Build history of the part. All positions in model axes, mm. A direction names the side the tool comes from. Give positions to 0.01 mm unless a question says otherwise; leave off trailing zeros. Loops run counter-clockwise (first coordinate to the right, second up) from the corner with the lowest first, then second, coordinate; pieces in that order, holes last. Notation, with made-up numbers: (27.5, 11.25) -> (52.5, 11.25) arc R28 cw to (52.5, 47.25) -> close; hole circle Ø6 at (53, 70.25). An arc over 180 degrees is marked (long way). Answer as a JSON object with one key per item and string values. Group by question number.
Q1. Two-plate mould, pull along X, no slides. Class faces 4 (the flat face through (0, 2, -13)), 5 (the cylindrical face through (-6.746, 7.1, -31.986)), 6 (the cylindrical face through (-0.1, 1, 6.5)): pulls with the +X half, pulls with the -X half, needs draft (parallel to the pull), parting line crosses it, or undercut.
Q2. Tool access for faces 1 (the flat face through (-6.5, 1, -16)), 2 (the flat face through (6.5, 1, -15)), 3 (the cylindrical face through (-7.14, 8.02, -31.99)): list every direction of +Z, -Z, +X, -X, +Y, -Y with a clear straight run to the whole face (end or side of a thin tool).
Q3. Band-saw the part on D-D, the plane x = -7.25. Write the cut outline in (y, z), plus the area to 3 significant figures.
Q4. Band-saw the part on C-C, the plane z = 1.5. Write the cut outline in (x, y).
Q5. Band-saw the part on B-B, the plane y = 13.5. Write the cut outline in (x, z).
Q6. Wall check: probe 1 along X at (y, z) = (0.6, 0); probe 2 along Y at (x, z) = (-7.7, -32.6); probe 3 along Z at (x, y) = (-3.25, 23.75). Give the ranges that are in metal, low to high. Write a range as from..to.
Q7. Drop flat-ended pins along their axis: pin 1 (2 mm diameter, centred on y = 1, z = -9.5, fed in from -X); pin 2 (1 mm diameter, centred on x = 0.5, y = 3.5, fed in from +Z); pin 3 (1.5 mm diameter, centred on x = -6.5, z = -3, fed in from +Y). Give the stop position or say it passes through.
Q8. Band-saw the part on A-A, the plane x = 0. Write the cut outline in (y, z), plus the area to 3 significant figures.
from build123d import *

# Parameters (mm, degrees)
SKETCH_2_R          = 6.5
EXTRUDE_1_DEPTH     = 2
SKETCH_3_R          = 2
CUT_EXTRUDE_2_DEPTH = 10.407443861
EXTRUDE_START       = -2
EXTRUDE_2_DEPTH     = 2
EXTRUDE_3_DEPTH     = 2
SKETCH_22_R         = 9
SKETCH_22_R_2       = 1
CUT_EXTRUDE_4_DEPTH = 2


with BuildPart() as part:
    # 草图2 → 凸台-拉伸1 (new body)
    with BuildSketch(Plane(origin=(0, 0, 0), x_dir=(1, 0, 0), z_dir=(0, 1, 0))):
        with Locations(Location((0, 0, 0), (0, 0, 270))):
            Circle(SKETCH_2_R)
    extrude(amount=EXTRUDE_1_DEPTH)

    # 草图3 → 切除-拉伸2 (cut, through all)
    with BuildSketch(Plane(origin=(0, 2, 0), x_dir=(1, 0, 0), z_dir=(0, 1, 0))):
        with Locations(Location((0, 0, 0), (0, 0, 270))):
            Circle(SKETCH_3_R)
    extrude(amount=-CUT_EXTRUDE_2_DEPTH, mode=Mode.SUBTRACT)

    # 草图4 → 凸台-拉伸2 (add)
    with BuildSketch(Plane(origin=(0, 2, 0), x_dir=(1, 0, 0), z_dir=(0, 1, 0)).offset(EXTRUDE_START)):
        with BuildLine():
            Line((6.5, 0), (6.5, 31))
            Line((6.5, 31), (3.899148682, 31))
            Line((3.899148682, 31), (-4.100851318, 31))
            Line((-4.100851318, 31), (-6.5, 31))
            Line((-6.5, 31), (-6.5, 0))
            ThreePointArc((-6.5, 0), (0, 6.5), (6.5, 0))
        make_face()
    extrude(amount=EXTRUDE_2_DEPTH)

    # 草图21 → 凸台-拉伸3 (add)
    with BuildSketch(Plane(origin=(0, 0, -31), x_dir=(-1, 0, 0), z_dir=(0, 0, -1))):
        Polygon((0, 0), (12, 0), (12, 25), (-12, 25), (-12, 0), align=None)
    extrude(amount=EXTRUDE_3_DEPTH)

    # 草图22 → 切除-拉伸4 (cut)
    with BuildSketch(Plane.XY.offset(-31)):
        with Locations((0, 13.5)):
            Circle(SKETCH_22_R)
        with Locations((7.7, 22.2)):
            Circle(SKETCH_22_R_2)
        with Locations((-7.7, 22.2)):
            Circle(SKETCH_22_R_2)
        with Locations((-7.7, 6.8)):
            Circle(SKETCH_22_R_2)
        with Locations((7.7, 6.8)):
            Circle(SKETCH_22_R_2)
    extrude(amount=-CUT_EXTRUDE_4_DEPTH, mode=Mode.SUBTRACT)


solid = part.part
Worked answers:
{
 "1": {"face 4": "needs draft", "face 5": "undercut", "face 6": "parting line crosses it"},
 "2": {"face 1": "+Z, -X, +Y, -Y", "face 2": "+Z, +X, +Y, -Y", "face 3": "+Z, -Z"},
 "3": {"outline": "(0, -33) -> (5.91, -33) -> (5.91, -31) -> (0, -31) -> close; (7.69, -33) -> (8.17, -33) -> (8.17, -31) -> (7.69, -31) -> close; (18.83, -33) -> (21.31, -33) -> (21.31, -31) -> (18.83, -31) -> close; (23.09, -33) -> (25, -33) -> (25, -31) -> (23.09, -31) -> close", "area": "21.5 mm2"},
 "4": {"outline": "(-6.32, 0) -> (-1.32, 0) -> (-1.32, 2) -> (-6.32, 2) -> close; (1.32, 0) -> (6.32, 0) -> (6.32, 2) -> (1.32, 2) -> close"},
 "5": {"outline": "(-12, -33) -> (-9, -33) -> (-9, -31) -> (-12, -31) -> close; (9, -33) -> (12, -33) -> (12, -31) -> (9, -31) -> close"},
 "6": {"probe 1": "-6.5..-2, 2..6.5", "probe 2": "0..5.8, 7.8..8.84, 18.16..21.2, 23.2..25", "probe 3": "-33..-31"},
 "7": {"pin 1": "x = -6.5", "pin 2": "z = -31", "pin 3": "y = 2"},
 "8": {"outline": "(0, -33) -> (4.5, -33) -> (4.5, -31) -> (2, -31) -> (2, -2) -> (0, -2) -> close; (0, 2) -> (2, 2) -> (2, 6.5) -> (0, 6.5) -> close; (22.5, -33) -> (25, -33) -> (25, -31) -> (22.5, -31) -> close", "area": "81.0 mm2"}
}
